Read the model definition and answer for the solid it produces. Units are mm, in the model's axes. Face numbers are marked on the shaded views. A direction names the side the tool comes from. Round coordinates to 2 decimals unless told otherwise and drop trailing zeros. Loops run counter-clockwise (first coordinate to the right, second up) from the corner with the lowest first, then second, coordinate; pieces in that order, holes last. Notation, with made-up numbers: (50, 69) - (109, 69) arc R31 ccw to (109, 106) - close; hole circle Ø7 at (22, 1.25). An arc over 180 degrees is marked (long way). Use CSV: the item, a comma, the result in double quotes. Start each with the question number.
1. Given pin 1 Ø3 at (x, z) = (1.5, 1) entering from +Y; pin 2 Ø2 at (x, y) = (1.5, -2) entering from +Z, each flat-ended and moving along its own axis, determine where each tip first touches the part or whether it passes through.
2. Find section B-B (y = -2.25). Give the vertices of the cut face in (x, z), and give its area (3 significant figures).
3. Consider line 1 along Y through (x, z) = (3.5, 0); line 2 along Y through (x, z) = (8, 0); line 3 along X through (y, z) = (-1.8, -1.95). Determine where each line is inside the solid, lowest interval first.
4. Find section A-A (x = 1). Give the vertices of the cut face in (y, z), and give its area (3 significant figures).
5. Determine the mould class of the marked faces 4, 5, 6 and 7 for opening direction X: +X half, -X half, draft (parallel to the pull), parting line (faces both ways), or undercut.
6. A tool of negligible diameter and unlimited length cuts with its end or side. For the marked faces 1, 2 and 3, from which of +Z, -Z, +X, -X, +Y, -Y can it reach the whole face along a straight path? Write none if from no direction.
7. Find section C-C (x = 5.25). Give the vertices of the cut face in (y, z).
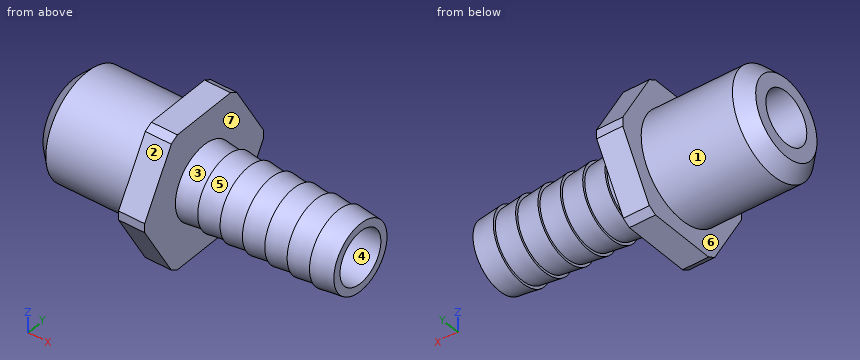
from build123d import *

# Parameters (mm, degrees)
CHAMFER1_SIZE      = 0.5
SKETCH2_R          = 6
CUT_EXTRUDE2_DEPTH = 9.185352772
CHAMFER2_SIZE      = 0.2


with BuildPart() as part:
    # Sketch1 → Revolve1 (revolve)
    with BuildSketch(Plane.XY, mode=Mode.PRIVATE) as revolve1_sk:
        Polygon((0, 1), (11, 1), (11, 1.3), (10.142857143, 1.4), (10.142857143, 1.3), (9.285714286, 1.4), (9.285714286, 1.3), (8.428571429, 1.4), (8.428571429, 1.3), (7.571428571, 1.4), (7.571428571, 1.3), (6.714285714, 1.4), (6.714285714, 1.3), (5.857142857, 1.4), (5.857142857, 1.3), (5, 1.4), (5, 3), (4, 3), (4, 2), (0, 2), align=None)
    revolve(revolve1_sk.sketch.rotate(Axis((0, 0, 0), (1, 0, 0)), 90), axis=Axis((0, 0, 0), (1, 0, 0)))

    # Chamfer1
    chamfer1_edges = [part.edges().sort_by_distance(p)[0] for p in [
        (0, 0, -2),
    ]]
    chamfer(chamfer1_edges, length=CHAMFER1_SIZE)

    # Sketch2 → Cut-Extrude2 (cut, through all)
    with BuildSketch(Plane.ZY.offset(-4)):
        Circle(SKETCH2_R)
        Polygon((0, 3), (-2.598076211, 1.5), (-2.598076211, -1.5), (0, -3), (2.598076211, -1.5), (2.598076211, 1.5), align=None, mode=Mode.SUBTRACT)
    extrude(amount=-CUT_EXTRUDE2_DEPTH, mode=Mode.SUBTRACT)

    # Chamfer2
    chamfer2_edges = [part.edges().sort_by_distance(p)[0] for p in [
        (4.5, 1.5, 2.598076211),
        (4.5, -1.5, 2.598076211),
        (4.5, -3, 0),
        (4.5, -1.5, -2.598076211),
        (4.5, 1.5, -2.598076211),
        (4.5, 3, 0),
    ]]
    chamfer(chamfer2_edges, length=CHAMFER2_SIZE)


solid = part.part
Filled sheet:
1,pin 1,"stops at y = 2"
1,pin 2,"stops at z = 1.73"
2,outline,"(4, -1.3) - (5, -1.3) - (5, 1.3) - (4, 1.3) - close"
2,area,"2.60 mm²"
3,line 1,"y = -2 to -1, 1 to 2"
3,line 2,"y = -1.35 to -1, 1 to 1.35"
3,line 3,"x = 4 to 5"
4,outline,"circle Ø4 at (0, 0); hole circle Ø2 at (0, 0)"
4,area,"9.42 mm²"
5,face 4,"draft"
5,face 5,"undercut"
5,face 6,"-X half"
5,face 7,"+X half"
6,face 1,"-X"
6,face 2,"+Z, +X, -X, -Y"
6,face 3,"none"
7,outline,"circle Ø2.74 at (0, 0); hole circle Ø2 at (0, 0)"
